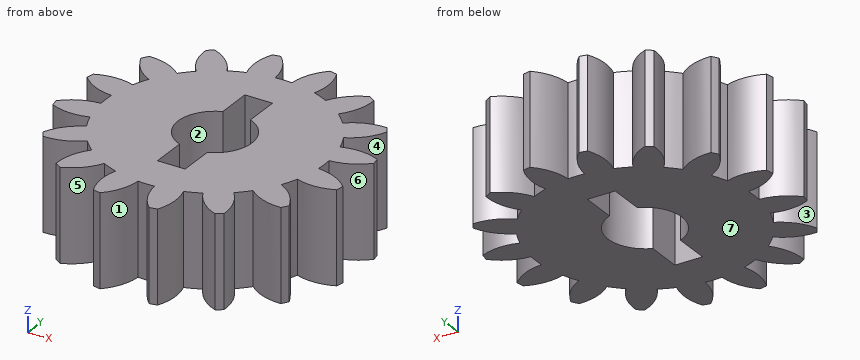
from build123d import *

# Parameters (mm, degrees)
BOSS_EXTRUDE1_DEPTH = 20


with BuildPart() as part:
    # Sketch1 → Boss-Extrude1 (new body)
    with BuildSketch(Plane.XY):
        with BuildLine():
            ThreePointArc((-31.046882255, 5.323636185), (-27.637166731, 2.849349951), (-23.55457664, 1.809777696))
            ThreePointArc((-23.55457664, 1.809777696), (-23.624, 0), (-23.55457664, -1.809777696))
            ThreePointArc((-23.55457664, -1.809777696), (-27.637166731, -2.849349951), (-31.046882255, -5.323636185))
            ThreePointArc((-31.046882255, -5.323636185), (-30.894736333, -6.145345143), (-30.720846432, -6.962728956))
            ThreePointArc((-30.720846432, -6.962728956), (-26.623811699, -7.943829725), (-22.454163195, -7.341929665))
            ThreePointArc((-22.454163195, -7.341929665), (-21.825730076, -9.040513406), (-21.069019314, -10.685962808))
            ThreePointArc((-21.069019314, -10.685962808), (-24.44301366, -13.208741926), (-26.646311696, -16.799525975))
            ThreePointArc((-26.646311696, -16.799525975), (-26.191292788, -17.50046234), (-25.717840224, -18.189081731))
            ThreePointArc((-25.717840224, -18.189081731), (-21.55722268, -17.527633336), (-17.935306952, -15.375894789))
            ThreePointArc((-17.935306952, -15.375894789), (-16.704690599, -16.704690599), (-15.375894789, -17.935306951))
            ThreePointArc((-15.375894789, -17.935306951), (-17.527633336, -21.55722268), (-18.189081731, -25.717840224))
            ThreePointArc((-18.189081731, -25.717840224), (-17.50046234, -26.191292788), (-16.799525975, -26.646311696))
            ThreePointArc((-16.799525975, -26.646311696), (-13.208741926, -24.44301366), (-10.685962808, -21.069019314))
            ThreePointArc((-10.685962808, -21.069019314), (-9.040513406, -21.825730076), (-7.341929665, -22.454163195))
            ThreePointArc((-7.341929665, -22.454163195), (-7.943829725, -26.623811699), (-6.962728956, -30.720846432))
            ThreePointArc((-6.962728956, -30.720846432), (-6.145345144, -30.894736333), (-5.323636185, -31.046882255))
            ThreePointArc((-5.323636185, -31.046882255), (-2.849349951, -27.637166731), (-1.809777696, -23.55457664))
            ThreePointArc((-1.809777696, -23.55457664), (0, -23.624), (1.809777696, -23.55457664))
            ThreePointArc((1.809777696, -23.55457664), (2.849349951, -27.637166731), (5.323636185, -31.046882255))
            ThreePointArc((5.323636185, -31.046882255), (6.145345143, -30.894736333), (6.962728956, -30.720846432))
            ThreePointArc((6.962728956, -30.720846432), (7.943829725, -26.623811699), (7.341929665, -22.454163195))
            ThreePointArc((7.341929665, -22.454163195), (9.040513406, -21.825730076), (10.685962808, -21.069019314))
            ThreePointArc((10.685962808, -21.069019314), (13.208741926, -24.44301366), (16.799525975, -26.646311696))
            ThreePointArc((16.799525975, -26.646311696), (17.50046234, -26.191292788), (18.189081731, -25.717840224))
            ThreePointArc((18.189081731, -25.717840224), (17.527633336, -21.55722268), (15.375894789, -17.935306952))
            ThreePointArc((15.375894789, -17.935306952), (16.704690599, -16.704690599), (17.935306952, -15.375894789))
            ThreePointArc((17.935306952, -15.375894789), (21.55722268, -17.527633336), (25.717840224, -18.189081731))
            ThreePointArc((25.717840224, -18.189081731), (26.191292788, -17.50046234), (26.646311696, -16.799525975))
            ThreePointArc((26.646311696, -16.799525975), (24.44301366, -13.208741926), (21.069019314, -10.685962808))
            ThreePointArc((21.069019314, -10.685962808), (21.825730076, -9.040513406), (22.454163195, -7.341929665))
            ThreePointArc((22.454163195, -7.341929665), (26.623811699, -7.943829725), (30.720846432, -6.962728956))
            ThreePointArc((30.720846432, -6.962728956), (30.894736333, -6.145345144), (31.046882255, -5.323636185))
            ThreePointArc((31.046882255, -5.323636185), (27.637166731, -2.849349951), (23.55457664, -1.809777696))
            ThreePointArc((23.55457664, -1.809777696), (23.624, 0), (23.55457664, 1.809777696))
            ThreePointArc((23.55457664, 1.809777696), (27.637166731, 2.849349951), (31.046882255, 5.323636185))
            ThreePointArc((31.046882255, 5.323636185), (30.894736333, 6.145345144), (30.720846432, 6.962728956))
            ThreePointArc((30.720846432, 6.962728956), (26.623811699, 7.943829725), (22.454163195, 7.341929665))
            ThreePointArc((22.454163195, 7.341929665), (21.825730076, 9.040513406), (21.069019314, 10.685962808))
            ThreePointArc((21.069019314, 10.685962808), (24.44301366, 13.208741926), (26.646311696, 16.799525975))
            ThreePointArc((26.646311696, 16.799525975), (26.191292788, 17.50046234), (25.717840224, 18.189081731))
            ThreePointArc((25.717840224, 18.189081731), (21.55722268, 17.527633336), (17.935306951, 15.375894789))
            ThreePointArc((17.935306951, 15.375894789), (16.704690599, 16.704690599), (15.375894789, 17.935306952))
            ThreePointArc((15.375894789, 17.935306952), (17.527633336, 21.55722268), (18.189081731, 25.717840224))
            ThreePointArc((18.189081731, 25.717840224), (17.50046234, 26.191292788), (16.799525975, 26.646311696))
            ThreePointArc((16.799525975, 26.646311696), (13.208741926, 24.44301366), (10.685962808, 21.069019314))
            ThreePointArc((10.685962808, 21.069019314), (9.040513406, 21.825730076), (7.341929665, 22.454163195))
            ThreePointArc((7.341929665, 22.454163195), (7.943829725, 26.623811699), (6.962728956, 30.720846432))
            ThreePointArc((6.962728956, 30.720846432), (6.145345144, 30.894736333), (5.323636185, 31.046882255))
            ThreePointArc((5.323636185, 31.046882255), (2.849349951, 27.637166731), (1.809777696, 23.55457664))
            ThreePointArc((1.809777696, 23.55457664), (0, 23.624), (-1.809777696, 23.55457664))
            ThreePointArc((-1.809777696, 23.55457664), (-2.849349951, 27.637166731), (-5.323636185, 31.046882255))
            ThreePointArc((-5.323636185, 31.046882255), (-6.145345144, 30.894736333), (-6.962728956, 30.720846432))
            ThreePointArc((-6.962728956, 30.720846432), (-7.943829725, 26.623811699), (-7.341929665, 22.454163195))
            ThreePointArc((-7.341929665, 22.454163195), (-9.040513406, 21.825730076), (-10.685962808, 21.069019314))
            ThreePointArc((-10.685962808, 21.069019314), (-13.208741926, 24.44301366), (-16.799525975, 26.646311696))
            ThreePointArc((-16.799525975, 26.646311696), (-17.50046234, 26.191292788), (-18.189081731, 25.717840224))
            ThreePointArc((-18.189081731, 25.717840224), (-17.527633336, 21.55722268), (-15.375894789, 17.935306952))
            ThreePointArc((-15.375894789, 17.935306952), (-16.704690599, 16.704690599), (-17.935306952, 15.375894789))
            ThreePointArc((-17.935306952, 15.375894789), (-21.55722268, 17.527633336), (-25.717840224, 18.189081731))
            ThreePointArc((-25.717840224, 18.189081731), (-26.191292788, 17.50046234), (-26.646311696, 16.799525975))
            ThreePointArc((-26.646311696, 16.799525975), (-24.44301366, 13.208741926), (-21.069019314, 10.685962808))
            ThreePointArc((-21.069019314, 10.685962808), (-21.825730076, 9.040513406), (-22.454163195, 7.341929665))
            ThreePointArc((-22.454163195, 7.341929665), (-26.623811699, 7.943829725), (-30.720846432, 6.962728956))
            ThreePointArc((-30.720846432, 6.962728956), (-30.894736333, 6.145345144), (-31.046882255, 5.323636185))
        make_face()
        with BuildLine():
            Line((-3, 15), (3, 15))
            Line((3, 15), (3, 7.416198487))
            ThreePointArc((3, 7.416198487), (8, 0), (3, -7.416198487))
            Line((3, -7.416198487), (3, -15))
            Line((3, -15), (-3, -15))
            Line((-3, -15), (-3, -7.416198487))
            ThreePointArc((-3, -7.416198487), (-8, 0), (-3, 7.416198487))
            Line((-3, 7.416198487), (-3, 15))
        make_face(mode=Mode.SUBTRACT)
    extrude(amount=BOSS_EXTRUDE1_DEPTH)


solid = part.part
Geometry check sheet. Reference: the model listing, model coordinates, mm. Face numbers are marked on the shaded views. A direction names the side the tool comes from. Round coordinates to 2 decimals unless told otherwise and drop trailing zeros. Loops run counter-clockwise (first coordinate to the right, second up) from the corner with the lowest first, then second, coordinate; pieces in that order, holes last. Notation, with made-up numbers: (79, 29.5) -> (133, 29.5) arc R21 ccw to (133, 60.5) -> close; hole circle Ø2 at (-4.5, -27.75). An arc over 180 degrees is marked (long way). Answer as a JSON object with one key per item and string values. Group by question number.
Item 1: Cross-section at C-C, the plane y = 0.5. Record the cut outline in (x, z), plus the area to 3 significant figures.
Item 2: Depth check by flat-ended pin: pin 1 Ø6 at (y, z) = (12.5, 13.5) entering from -X; pin 2 Ø5 at (y, z) = (-12.5, 14.5) entering from +X; pin 3 Ø6 at (y, z) = (-23, 3) entering from -X; pin 4 Ø1.5 at (x, y) = (-14.5, -5.5) entering from -Z. Enter the tip coordinate at first touch or a pass-through.
Item 3: Release check for a two-part mould opening along Y. For the marked faces 5, 6 and 7 record: pulls with the +Y half, pulls with the -Y half, needs draft (parallel to the pull), parting line crosses it, or undercut.
Item 4: Set-up check for the marked faces 1, 2, 3 and 4: record each of +Z, -Z, +X, -X, +Y, -Y from which the full face is reachable in a straight line by a thin tool's end or side.
Item 5: Thickness scan on line 1 along Y through (x, z) = (-17, 6); line 2 along X through (y, z) = (-16, 10); line 3 along X through (y, z) = (-26.5, 12). Record the ranges inside material, lowest first.
Item 6: Cross-section at A-A, the plane y = -12. Record the cut outline in (x, z), plus the area to 3 significant figures.
Item 7: Cross-section at B-B, the plane y = -24.5. Record the cut outline in (x, z).
Determined:
{
 "1": {"outline": "(-23.62, 0) -> (-7.98, 0) -> (-7.98, 20) -> (-23.62, 20) -> close; (7.98, 0) -> (23.62, 0) -> (23.62, 20) -> (7.98, 20) -> close", "area": "625 mm²"},
 "2": {"pin 1": "stops at x = -26.06", "pin 2": "stops at x = 25.78", "pin 3": "stops at x = -18.19", "pin 4": "stops at z = 0"},
 "3": {"face 5": "pulls with the -Y half", "face 6": "undercut", "face 7": "needs draft"},
 "4": {"face 1": "+Z, -Z, -Y", "face 2": "+Z, -Z", "face 3": "+Z, -Z, -X", "face 4": "+Z, -Z, +X"},
 "5": {"line 1": "y = -26.52 to -20.33, -16.4 to 16.4, 20.33 to 26.52", "line 2": "x = -26.31 to -18.71, -17.38 to 17.38, 18.71 to 26.31", "line 3": "x = -17.03 to -16.43, -7.95 to -2.39, 2.39 to 7.95, 16.43 to 17.03"},
 "6": {"outline": "(-23.15, 0) -> (-3, 0) -> (-3, 20) -> (-23.15, 20) -> close; (3, 0) -> (23.15, 0) -> (23.15, 20) -> (3, 20) -> close", "area": "806 mm²"},
 "7": {"outline": "(-18.16, 0) -> (-13.27, 0) -> (-13.27, 20) -> (-18.16, 20) -> close; (-7.84, 0) -> (-1.91, 0) -> (-1.91, 20) -> (-7.84, 20) -> close; (1.91, 0) -> (7.84, 0) -> (7.84, 20) -> (1.91, 20) -> close; (13.27, 0) -> (18.16, 0) -> (18.16, 20) -> (13.27, 20) -> close"}
}
